Build history of the part. All positions in model axes, mm. Face numbers are marked on the shaded views. A direction names the side the tool comes from. Round coordinates to 2 decimals unless told otherwise and drop trailing zeros. Order: outer loops, then holes, each group sorted by start corner. A loop starts at its lowest first (then second) coordinate and runs counter-clockwise, first axis right, second up. Notation, with made-up numbers: M -21.5,31.5 L 36.5,31.5 A16 ccw 36.5,38.5 Z; hole C 45.25,-0.5 d3. An arc over 180 degrees is marked long. Use CSV: the item, a comma, the result in double quotes.
from build123d import *

# Parameters (mm, degrees)
SKETCH2_R           = 25.5
SKETCH2_R_2         = 15.5
BOSS_EXTRUDE1_DEPTH = 70
SKETCH3_R           = 17.5
CUT_EXTRUDE1_DEPTH  = 10
SKETCH4_R           = 17.5
CUT_EXTRUDE2_DEPTH  = 10
FILLET1_R           = 1


with BuildPart() as part:
    # Sketch2 → Boss-Extrude1 (new body)
    with BuildSketch(Plane(origin=(0, 0, 0), x_dir=(0, 0, -1), z_dir=(1, 0, 0))):
        Circle(SKETCH2_R)
        Circle(SKETCH2_R_2, mode=Mode.SUBTRACT)
    extrude(amount=BOSS_EXTRUDE1_DEPTH)

    # Sketch3 → Cut-Extrude1 (cut)
    with BuildSketch(Plane(origin=(70, 0, 0), x_dir=(0, 0, -1), z_dir=(1, 0, 0))):
        Circle(SKETCH3_R)
    extrude(amount=-CUT_EXTRUDE1_DEPTH, mode=Mode.SUBTRACT)

    # Sketch4 → Cut-Extrude2 (cut)
    with BuildSketch(Plane.ZY):
        Circle(SKETCH4_R)
    extrude(amount=-CUT_EXTRUDE2_DEPTH, mode=Mode.SUBTRACT)

    # Fillet1
    fillet1_edges = [part.edges().sort_by_distance(p)[0] for p in [
        (70, 0, 17.5),
        (0, 0, -17.5),
        (0, 0, 25.5),
        (70, 0, 25.5),
    ]]
    fillet(fillet1_edges, radius=FILLET1_R)


solid = part.part
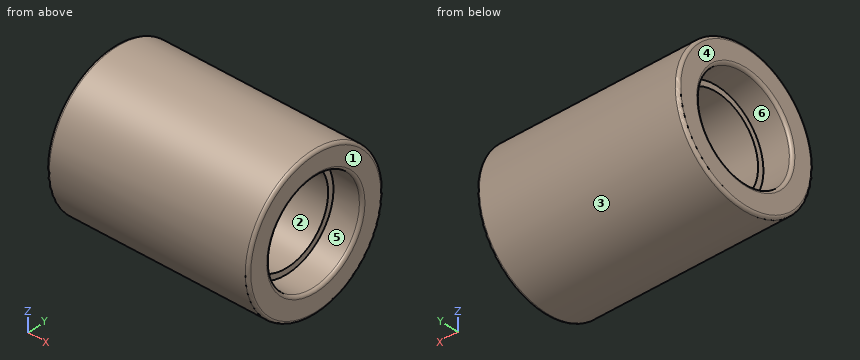
(1) Cut at A-A, the plane y = 0. Give the cut face in (x, z).
Answer block:
outline,"M 0,-24.5 A1 ccw 1,-25.5 L 69,-25.5 A1 ccw 70,-24.5 L 70,-18.5 A1 ccw 69,-17.5 L 60,-17.5 L 60,-15.5 L 10,-15.5 L 10,-17.5 L 1,-17.5 A1 ccw 0,-18.5 Z; M 0,18.5 A1 ccw 1,17.5 L 10,17.5 L 10,15.5 L 60,15.5 L 60,17.5 L 69,17.5 A1 ccw 70,18.5 L 70,24.5 A1 ccw 69,25.5 L 1,25.5 A1 ccw 0,24.5 Z"
(2) Cut at C-C, the plane x = 5. Give the cut face in (y, z).
Answer block:
outline,"C 0,0 d51; hole C 0,0 d35"
(3) Wall check: line 1 (Y direction, x = 66.75, z = 0); line 2 (Y direction, x = 22, z = 0); line 3 (Z direction, x = 56, y = 0.5). Give the ranges that are in metal, low to high. Write a range as from..to.
Answer block:
line 1,"y = -25.5..-17.5, 17.5..25.5"
line 2,"y = -25.5..-15.5, 15.5..25.5"
line 3,"z = -25.5..-15.49, 15.49..25.5"
(4) Tool access for the marked faces 4, 5 and 6: list every direction of +Z, -Z, +X, -X, +Y, -Y with a clear straight run to the whole face (end or side of a thin tool).
Answer block:
face 4,"+Z, -Z, -X, +Y, -Y"
face 5,"+X"
face 6,"-X"
(5) Cut at D-D, the plane x = 51. Give the cut face in (y, z), and give its area (3 significant figures).
Answer block:
outline,"C 0,0 d51; hole C 0,0 d31"
area,"1,290 mm²"
(6) Two-plate mould, pull along Z, no slides. Class the marked faces 1, 2 and 3: released by +Z, released by -Z, zero draft, split by the parting line, or undercut.
Answer block:
face 1,"zero draft"
face 2,"undercut"
face 3,"split by the parting line"
(7) Drop flat-ended pins along their axis: pin 1 (12 mm diameter, centred on x = 14, z = 10, fed in from -Y); pin 2 (8 mm diameter, centred on x = 31.5, y = 9, fed in from -Z) (3 decimals); pin 3 (12 mm diameter, centred on x = 49, y = 16.5, fed in from +Z); pin 4 (18.5 mm diameter, centred on y = 0, z = 0, fed in from -X). Give the stop position or say it passes through.
Answer block:
pin 1,"stops at y = -25.18"
pin 2,"stops at z = -25.005"
pin 3,"stops at z = 23.24"
pin 4,"passes through"
